```python
from build123d import *

# Parameters (mm, degrees)
F0_R     = 2.8
F0_W     = 8
F0_H     = 0.45
F1_DEPTH = 24
F2_R     = 1.95
F3_DEPTH = 9.951
F4_W     = 7.4
F4_H     = 3.5
F5_DEPTH = 12
F7_DEPTH = 3.5


# Not quite as in the source:
# - a feature names something its author has since deleted; it is built from what else it names


with BuildPart() as f1:
    # F0 (on Top) → F1 (new body)
    with BuildSketch(Plane.XY):
        with BuildLine():
            ThreePointArc((-8, 2.8), (-5.2, 0), (-8, -2.8))
            Line((-8, -2.8), (-12.75, -2.8))
            Line((-12.75, -2.8), (-12.75, -4.75))
            Line((-12.75, -4.75), (-8, -4.75))
            Line((-8, -4.75), (-4, -4.75))
            Line((-4, -4.75), (-4, -4.3))
            Line((-4, -4.3), (4, -4.3))
            Line((4, -4.3), (4, -4.75))
            Line((4, -4.75), (8, -4.75))
            ThreePointArc((8, -4.75), (12.75, 0), (8, 4.75))
            Line((8, 4.75), (-8, 4.75))
            Line((-8, 4.75), (-12.75, 4.75))
            Line((-12.75, 4.75), (-12.75, 2.8))
            Line((-12.75, 2.8), (-8, 2.8))
        make_face()
        with Locations((8, 0)):
            Circle(F0_R, mode=Mode.SUBTRACT)
        with Locations((0, -4.525)):
            Rectangle(F0_W, F0_H)
        with Locations((0, -4.975)):
            Rectangle(F0_W, F0_H)
    extrude(amount=F1_DEPTH)

    # F2 (on face) → F3 (cut, through all)
    with BuildSketch(Plane.XZ.offset(5.2)):
        with Locations((0, 12)):
            Circle(F2_R)
    extrude(amount=-F3_DEPTH, mode=Mode.SUBTRACT)

    # F4 (on face) → F5 (cut)
    with BuildSketch(Plane.XY.offset(24)):
        Rectangle(F4_W, F4_H)
    extrude(amount=-F5_DEPTH, mode=Mode.SUBTRACT)

    # F6 (on face) → F7 (cut, through all)
    with BuildSketch(Plane.XZ.offset(-1.75)):
        Polygon((3.7, 9.563804004), (3.7, 13.836195996), (0, 15.972391992), (-3.7, 13.836195996), (-3.7, 9.563804004), (0, 7.427608008), align=None)
    extrude(amount=F7_DEPTH, mode=Mode.SUBTRACT)


solid = f1.part
```
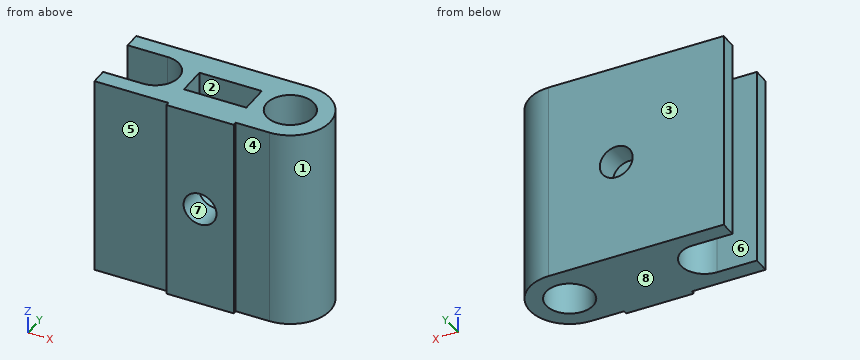
Check sheet for the modelled part. Datum: model origin and axes. Units: mm. Face numbers are marked on the shaded views. A direction names the side the tool comes from. Give positions to 0.01 mm unless a question says otherwise; leave off trailing zeros. Order: outer loops, then holes, each group sorted by start corner. A loop starts at its lowest first (then second) coordinate and runs counter-clockwise, first axis right, second up. Notation, with made-up numbers: M 19.5,-3.75 L 73.5,-3.75 A32 ccw 73.5,24.25 Z; hole C 60.5,-4 d3. An arc over 180 degrees is marked long. Answer in a Markdown table with one row per item.
1) Cross-section at B-B, the plane x = -10. Enter the section's corners in (y, z).
Filled sheet:
| item | result |
|---|---|
| outline | M -4.75,0 L -2.8,0 L -2.8,24 L -4.75,24 Z; M 2.8,0 L 4.75,0 L 4.75,24 L 2.8,24 Z |
2) Access from +Z, -Z, +X, -X, +Y, -Y to the whole of each face (thin tool, end or side, straight path). Record for the marked faces 4, 5, 6, 7 and 8.
Filled sheet:
| item | result |
|---|---|
| face 4 | +Z, -Z, +X, -Y |
| face 5 | +Z, -Z, -X, -Y |
| face 6 | +Z, -Z, -X |
| face 7 | +Y, -Y |
| face 8 | -Z, +X, -X, +Y, -Y |
3) Gauge pin test, flat ends, axial feed: P1, Ø4, axis at x = -11, z = 9, coming from the -Y side; P2, Ø5, axis at y = -1.5, z = 5, coming from the +X side; P3, Ø1.8, axis at y = -1, z = 15.5, coming from the -X side; P4, Ø2, axis at y = -2, z = 18.5, coming from the +X side. Record the tip position at first contact, or that the pin passes through.
Filled sheet:
| item | result |
|---|---|
| P1 | stops at y = -4.75 |
| P2 | stops at x = 12.75 |
| P3 | stops at x = -5.94 |
| P4 | stops at x = 12.64 |
4) Thickness scan on L1, parallel to Y at x = -9.75, z = 9; L2, parallel to X at y = 2, z = 13.75; L3, parallel to Y at x = -1, z = 17.5. Record the ranges inside material, lowest first. Write a range as [from, to].
Filled sheet:
| item | result |
|---|---|
| L1 | y = [-4.75, -2.8], [2.8, 4.75] |
| L2 | x = [-6.04, -0.86], [0.86, 6.04], [9.96, 12.31] |
| L3 | y = [-5.2, -1.75], [1.75, 4.75] |
5) Release check for a two-part mould opening along X. For the marked faces 1, 2 and 3 record: +X half, -X half, draft (parallel to the pull), parting line (faces both ways), or undercut.
Filled sheet:
| item | result |
|---|---|
| face 1 | +X half |
| face 2 | undercut |
| face 3 | draft |
6) Cross-section at A-A, the plane z = 12. Enter the section's corners in (x, y), plus the area to 3 significant figures.
Filled sheet:
| item | result |
|---|---|
| outline | M -12.75,-4.75 L -4,-4.75 L -4,-5.2 L -1.95,-5.2 L -1.95,-1.75 L -3.7,-1.75 L -3.7,1.75 L -1.95,1.75 L -1.95,4.75 L -12.75,4.75 L -12.75,2.8 L -8,2.8 A2.8 cw -8,-2.8 L -12.75,-2.8 Z; M 1.95,-5.2 L 4,-5.2 L 4,-4.75 L 8,-4.75 A4.75 ccw 8,4.75 L 1.95,4.75 L 1.95,1.75 L 3.7,1.75 L 3.7,-1.75 L 1.95,-1.75 Z; hole C 8,0 d5.6 |
| area | 122 mm2 |
7) Cross-section at D-D, the plane z = 2.25. Enter the section's corners in (x, y).
Filled sheet:
| item | result |
|---|---|
| outline | M -12.75,-4.75 L -4,-4.75 L -4,-5.2 L 4,-5.2 L 4,-4.75 L 8,-4.75 A4.75 ccw 8,4.75 L -12.75,4.75 L -12.75,2.8 L -8,2.8 A2.8 cw -8,-2.8 L -12.75,-2.8 Z; hole C 8,0 d5.6 |
8) Cross-section at C-C, the plane y = 0. Enter the section's corners in (x, z), plus the area to 3 significant figures.
Filled sheet:
| item | result |
|---|---|
| outline | M -5.2,0 L 5.2,0 L 5.2,24 L 3.7,24 L 3.7,9.56 L 0,7.43 L -3.7,9.56 L -3.7,24 L -5.2,24 Z; M 10.8,0 L 12.75,0 L 12.75,24 L 10.8,24 Z |
| area | 182 mm2 |
